Verification items for the finished model (mm, model axes). Face numbers are marked on the shaded views. A direction names the side the tool comes from. Give positions to 0.01 mm unless a question says otherwise; leave off trailing zeros. Write each loop counter-clockwise with the first axis right and the second up, starting at its lowest first coordinate (ties: lowest second). Pieces come first, ordered by that corner, then holes. Notation, with made-up numbers: (24, 32) -> (83, 32) arc R34 cw to (83, 66) -> close; hole circle Ø2 at (68.25, 67.25). An arc over 180 degrees is marked (long way). Use one line per item in the form item = value. Start each with the question number.
(1) Release check for a two-part mould opening along Y. For the marked faces 3, 4, 5 and 6 record: pulls with the +Y half, pulls with the -Y half, needs draft (parallel to the pull), parting line crosses it, or undercut.
(2) Section check C-C, the plane y = 34. Record the cut outline in (x, z), plus the area to 3 significant figures.
(3) Depth check by flat-ended pin: pin 1 Ø1 at (x, y) = (5.5, -10.5) entering from -Z; pin 2 Ø1.5 at (y, z) = (35, 1) entering from +X. Enter the tip coordinate at first touch or a pass-through.
(4) Section check D-D, the plane x = 9.25. Record the cut outline in (y, z), plus the area to 3 significant figures.
(5) Set-up check for the marked faces 1 and 2: record each of +Z, -Z, +X, -X, +Y, -Y from which the full face is reachable in a straight line by a thin tool's end or side.
(6) Section check B-B, the plane x = 6.25. Record the cut outline in (y, z), plus the area to 3 significant figures.
(7) Section check A-A, the plane z = 1.35. Record the cut outline in (x, y), plus the area to 3 significant figures.
(8) Scan lines: L1, parallel to X at y = 34.5, z = 1.1; L2, parallel to X at y = 26, z = 0.25. Record each from-to range of solid material in increasing order.
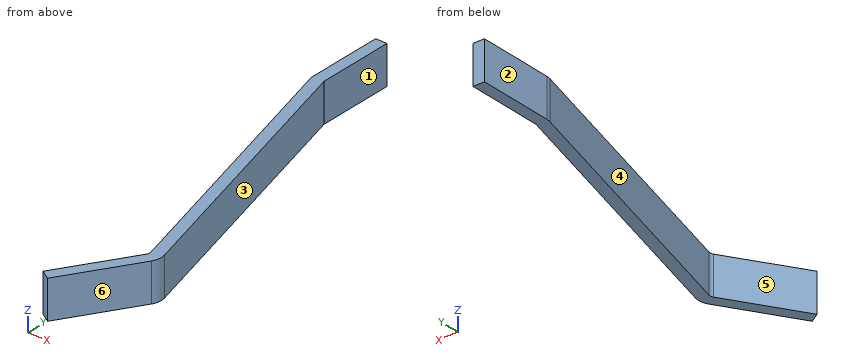
from build123d import *

# Parameters (mm, degrees)
BASE_FLANGE1_DEPTH      = 2.5
BASE_FLANGE1_DEPTH_BACK = 2.5


# Sheet-metal steps are written as plain solids
with BuildPart() as part:
    # Sketch1 → Base-Flange1 (new, two sides: drawn at the far end of the back side and taken through both)
    with BuildSketch(Plane.XY.offset(-BASE_FLANGE1_DEPTH_BACK)):
        with BuildLine():
            Line((0, 39.604011434), (0, 29.700986664))
            ThreePointArc((0, 29.700986664), (0.006301715, 29.60484107), (0.025099036, 29.510340555))
            Line((0.025099036, 29.510340555), (10.101059931, -8.09365744))
            ThreePointArc((10.101059931, -8.09365744), (10.152703108, -9.003122645), (9.8374146, -9.857749543))
            Line((9.8374146, -9.857749543), (3.993730633, -19.209598772))
            Line((3.993730633, -19.209598772), (2.721658489, -18.414719875))
            Line((2.721658489, -18.414719875), (8.565342456, -9.062870646))
            ThreePointArc((8.565342456, -9.062870646), (8.669179313, -8.781408529), (8.652171192, -8.481886008))
            Line((8.652171192, -8.481886008), (-1.423789703, 29.122111987))
            ThreePointArc((-1.423789703, 29.122111987), (-1.480865577, 29.409051782), (-1.5, 29.700986664))
            Line((-1.5, 29.700986664), (-1.5, 39.604011434))
            Line((-1.5, 39.604011434), (0, 39.604011434))
        make_face()
    extrude(amount=BASE_FLANGE1_DEPTH + BASE_FLANGE1_DEPTH_BACK)


solid = part.part
Completed:
q1.face_3 = pulls with the +Y half
q1.face_4 = undercut
q1.face_5 = undercut
q1.face_6 = pulls with the -Y half
q2.outline = (-1.5, -2.5) -> (0, -2.5) -> (0, 2.5) -> (-1.5, 2.5) -> close
q2.area = 7.50 mm²
q3.pin_1 = through
q3.pin_2 = 0
q4.outline = (-10.8, -2.5) -> (-4.92, -2.5) -> (-4.92, 2.5) -> (-10.8, 2.5) -> close
q4.area = 29.4 mm²
q5.face_1 = +Z, -Z, +X, +Y
q5.face_2 = +Z, -Z, -X, +Y, -Y
q6.outline = (-15.6, -2.5) -> (-12.77, -2.5) -> (-12.77, 2.5) -> (-15.6, 2.5) -> close; (0.48, -2.5) -> (6.28, -2.5) -> (6.28, 2.5) -> (0.48, 2.5) -> close
q6.area = 43.1 mm²
q7.outline = (-1.5, 29.7) arc R2.24 ccw to (-1.42, 29.12) -> (8.65, -8.48) arc R0.74 cw to (8.57, -9.06) -> (2.72, -18.41) -> (3.99, -19.21) -> (9.84, -9.86) arc R2.24 ccw to (10.1, -8.09) -> (0.03, 29.51) arc R0.74 cw to (0, 29.7) -> (0, 39.6) -> (-1.5, 39.6) -> close
q7.area = 92.2 mm²
q8.L1 = -1.5 to 0
q8.L2 = -0.59 to 0.97
